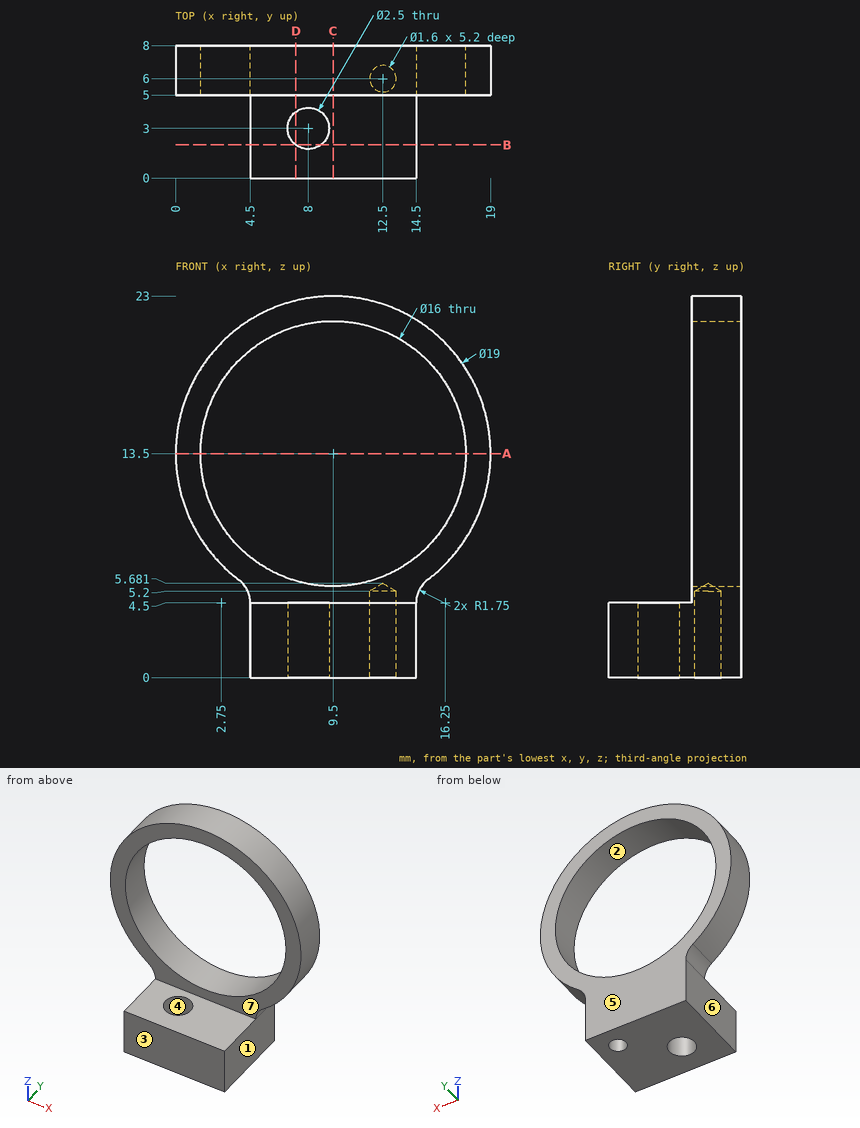
The drawing under review shows one solid part. Ordinate dimensions are in mm from its lowest x, y, z. A direction names the side the tool comes from. Give positions to 0.01 mm unless a question says otherwise; leave off trailing zeros. Write each loop counter-clockwise with the first axis right and the second up, starting at its lowest first coordinate (ties: lowest second). Pieces come first, ordered by that corner, then holes.
1. Add section C-C, the plane x = 9.5. Write out the cut boundary in (y, z).
2. Tool access review of the marked faces 5, 6 and 7: name each direction out of +Z, -Z, +X, -X, +Y, -Y from which nothing blocks a thin tool from reaching the whole face with its end or side.
3. Draft analysis for pull direction X (two halves, no side actions). For the marked faces 1, 2, 3 and 4, state which applies: +X half, -X half, draft (parallel to the pull), parting line (faces both ways), or undercut.
4. Add section D-D, the plane x = 7.25. Write out the cut boundary in (y, z).
5. Wall thickness on L1, parallel to Y at x = 12.5, z = 4.15; L2, parallel to X at y = 6, z = 2.5; L3, parallel to Y at x = 8, z = 3.05: over which ranges is each line inside the solid? List them lowest first.
6. Add section A-A, the plane z = 13.5. Write out the cut boundary in (x, y).
7. For P1, Ø4, axis at x = 8, y = 3, coming from the -Z side; P2, Ø1.5, axis at x = 12.5, y = 5, coming from the +Z side; P3, Ø2.5, axis at y = 3, z = 3, coming from the -X side; P4, Ø3, axis at y = 4.5, z = 18.5, coming from the +X side, all flat-tipped, find the tip position at first contact; note any pin that passes through.
8. Add section B-B, the plane y = 2. Write out the cut boundary in (x, z).
Worked answers:
1. outline: (0, 0) - (8, 0) - (8, 5.5) - (5, 5.5) - (5, 4.5) - (0, 4.5) - close; (5, 21.5) - (8, 21.5) - (8, 23) - (5, 23) - close
2. face 5: +Z, -Z, +X, -X, +Y
2. face 6: -Z, -X, +Y, -Y
2. face 7: +Z, +X, -X, -Y
3. face 1: +X half
3. face 2: undercut
3. face 3: draft
3. face 4: undercut
4. outline: (0, 0) - (2, 0) - (2, 4.5) - (0, 4.5) - close; (4, 0) - (8, 0) - (8, 5.82) - (5, 5.82) - (5, 4.5) - (4, 4.5) - close; (5, 21.18) - (8, 21.18) - (8, 22.73) - (5, 22.73) - close
5. L1: y = 0 to 5.2, 6.8 to 8
5. L2: x = 4.5 to 11.7, 13.3 to 14.5
5. L3: y = 0 to 1.75, 4.25 to 8
6. outline: (0, 5) - (1.5, 5) - (1.5, 8) - (0, 8) - close; (17.5, 5) - (19, 5) - (19, 8) - (17.5, 8) - close
7. P1: stops at z = 0
7. P2: stops at z = 22.73
7. P3: stops at x = 4.5
7. P4: stops at x = 18.3
8. outline: (4.5, 0) - (7.25, 0) - (7.25, 4.5) - (4.5, 4.5) - close; (8.75, 0) - (14.5, 0) - (14.5, 4.5) - (8.75, 4.5) - close
